Can you work these out from the model? Positions are in its coordinate system, mm. A direction names the side the tool comes from. Round coordinates to 2 decimals unless told otherwise and drop trailing zeros. Order: outer loops, then holes, each group sorted by start corner. A loop starts at its lowest first (then second) coordinate and runs counter-clockwise, first axis right, second up.
Autodesk Inventor part; units mm, degrees
ref_plane "YZ Plane" through (0, 0, 0) normal (1, 0, 0) x (0, 1, 0)
ref_plane "XZ Plane" through (0, 0, 0) normal (0, 1, 0) x (-1, 0, 0)
ref_plane "XY Plane" through (0, 0, 0) normal (0, 0, 1) x (1, 0, 0)
sketch "Sketch1" plane through (0, 0, 0) normal (0, 0, 1) x (1, 0, 0)
  line L0 (-346.0753, 70.9014) -> (-181.3844, 70.9014) construction
  line L1 (-181.3844, 70.9014) -> (-181.3844, -72.4094) construction
  line L2 (-181.3844, -72.4094) -> (-346.0753, -72.4094) construction
  line L3 (-346.0753, -72.4094) -> (-346.0753, 70.9014) construction
  line L4 (25, 32.5) -> (25, -32.5)
  line L5 (-25, -32.5) -> (-25, 32.5)
  line L6 (-25, 32.5) -> (25, -32.5) construction
  line L7 (25, 32.5) -> (-25, -32.5) construction
  line L8 (15, -2.5) -> (-15, -2.5)
  arc A0 (-25, 32.5) -> (25, 32.5) centre (0, 32.5) ccw
  line L9 (-25, -32.5) -> (-55, -32.5)
  line L10 (-55, -32.5) -> (-55, -77.5)
  line L11 (-55, -77.5) -> (-45, -77.5)
  line L12 (-45, -77.5) -> (-45, -42.5)
  line L13 (25, -32.5) -> (55, -32.5)
  line L14 (55, -32.5) -> (55, -77.5)
  line L15 (55, -77.5) -> (45, -77.5)
  line L16 (45, -77.5) -> (45, -42.5)
  line L17 (-15, -2.5) -> (-15, -42.5)
  line L18 (15, -2.5) -> (15, -42.5)
  line L19 (-45, -42.5) -> (-15, -42.5)
  line L20 (15, -42.5) -> (45, -42.5)
  point P0 (0, 0)
  dimension "d3" = 50
  dimension "d4" = 65
  dimension "d15" = 25
  dimension "d16" = 90
  dimension "d18" = 30
  dimension "d19" = 45
extrude "Extrusion1" add sketch "Sketch1" along normal blind 40
sketch "Sketch2" plane through (0, 0, 40) normal (0, 0, 1) x (1, 0, 0)
  arc A0 (-25, 32.5) -> (25, 32.5) centre (0, 32.5) ccw
  circle A1 centre (0, 32.5) radius 25
  point P0 (0, 0)
  point P1 (25, 32.5)
  dimension "d26" = 50
extrude "Extrusion2" add sketch "Sketch2" along normal blind 30 and the other way blind 50
sketch "Sketch3" plane through (0, 32.5, 70) normal (0, 0, 1) x (1, 0, 0)
  arc A0 (-25, 0) -> (25, 0) centre (0, 0) ccw
  circle A1 centre (0, 0) radius 17.5
  circle A2 centre (0, 0) radius 10
  point P0 (0, -32.5)
  dimension "d31" = 35
  dimension "d32" = 20
extrude "Extrusion3" add sketch "Sketch3" along normal blind 16
sketch "Sketch4" plane through (45, -77.5, 0) normal (0, -1, 0) x (1, 0, 0)
  point P0 (-45, 0)
sketch "Sketch5" plane through (55, -77.5, 0) normal (1, 0, 0) x (0, 0, -1)
  circle A0 centre (-20, 21.3987) radius 12
  line L0 (0, 0) -> (0, 45)
  point P0 (0, 77.5)
  dimension "d35" = 24
  dimension "d36" = 20
extrude "Extrusion4" cut sketch "Sketch5" against normal blind 120
properties part number "cad@54"
(1) On a 3-axis mill with a long thin cutter (end or side, diameter ignored), from which of +Z, -Z, +X, -X, +Y, -Y can I reach the whole of each face in a straight line? I mean faces 1 (the face through (45, -68, 15)), 2 (the face through (40, -32.5, 20)), 3 (the face through (-40, -32.5, 20)). Say none if no direction works.
(2) I'm going to push flat-ended pins straight in: pin 1 Ø1.5 at (y, z) = (30.5, 76) entering from -X; pin 2 Ø12 at (y, z) = (-9, 42) entering from +X; pin 3 Ø15 at (x, z) = (-45, 13) entering from +Y; pin 4 Ø2 at (x, y) = (-27, 36.5) entering from -Z. Where does each tip first touch, or does it pass through?
(3) I want a section at D-D, the plane z = 4. List the corners of the cut face in (x, y) for me.
(4) I want a section at A-A, the plane z = 20. List the corners of the cut face in (x, y) for me.
(5) I want a section at B-B, the plane y = -23.5. List the corners of the cut face in (x, z) for me.
(6) Please list where these lines run through material, in increasing order: probe 1 along X at (y, z) = (-69.5, 12.5); probe 2 along Y at (x, z) = (0, 79.5); probe 3 along Y at (x, z) = (28.5, 17).
(7) I want a section at C-C, the plane x = 0. List the corners of the cut face in (y, z) for me, plus the area to 3 significant figures.
(8) If we mould it in two halves opening along Y, with no side actions, what happens to faces 4 (the face through (-12.898, 20.673, 77.888)), 5 (the face through (5, 50, 70)), 6 (the face through (0, 33, 70))? For each: pulls with the +Y half, pulls with the -Y half, needs draft (parallel to the pull), parting line crosses it, or undercut.
Ans:
1. face 1: +Z, -Z, -Y
1. face 2: +Z, -Z, +X, +Y
1. face 3: +Z, -Z, -X, +Y
2. pin 1: stops at x = -17.46
2. pin 2: stops at x = 25
2. pin 3: stops at y = -32.5
2. pin 4: passes through
3. outline: (-55, -77.5) - (-45, -77.5) - (-45, -42.5) - (-15, -42.5) - (-15, -2.5) - (15, -2.5) - (15, -42.5) - (45, -42.5) - (45, -77.5) - (55, -77.5) - (55, -32.5) - (25, -32.5) - (25, 32.5) arc R25 ccw to (-25, 32.5) - (-25, -32.5) - (-55, -32.5) - close
4. outline: (-55, -77.5) - (-45, -77.5) - (-45, -68.1) - (-55, -68.1) - close; (-55, -44.1) - (-45, -44.1) - (-45, -42.5) - (-15, -42.5) - (-15, -2.5) - (15, -2.5) - (15, -42.5) - (45, -42.5) - (45, -44.1) - (55, -44.1) - (55, -32.5) - (25, -32.5) - (25, 32.5) arc R25 ccw to (-25, 32.5) - (-25, -32.5) - (-55, -32.5) - close; (45, -77.5) - (55, -77.5) - (55, -68.1) - (45, -68.1) - close
5. outline: (-25, 0) - (-15, 0) - (-15, 40) - (-25, 40) - close; (15, 0) - (25, 0) - (25, 40) - (15, 40) - close
6. probe 1: x = -55 to -45, 45 to 55
6. probe 2: y = 15 to 22.5, 42.5 to 50
6. probe 3: y = -42.5 to -32.5
7. outline: (-2.5, 0) - (7.5, 0) - (7.5, -10) - (57.5, -10) - (57.5, 70) - (50, 70) - (50, 86) - (42.5, 86) - (42.5, 70) - (22.5, 70) - (22.5, 86) - (15, 86) - (15, 70) - (7.5, 70) - (7.5, 40) - (-2.5, 40) - close
7. area: 4,640 mm2
8. face 4: parting line crosses it
8. face 5: needs draft
8. face 6: undercut
